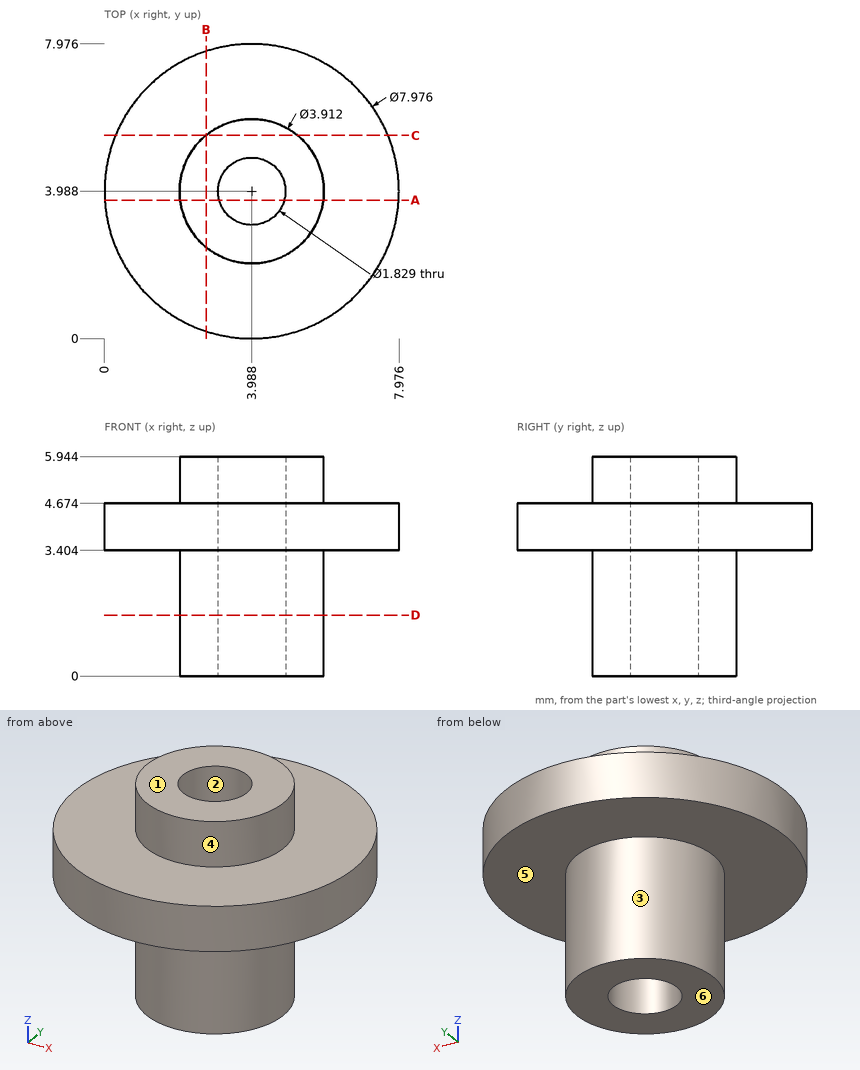
Part print with two shaded views. Sizes in mm from the minimum x, y, z corner. A direction names the side the tool comes from. Round coordinates to 2 decimals unless told otherwise and drop trailing zeros. Order: outer loops, then holes, each group sorted by start corner. A loop starts at its lowest first (then second) coordinate and runs counter-clockwise, first axis right, second up. Notation, with made-up numbers: (-12.75, 41) - (18.25, 41) arc R28 ccw to (18.25, 74) - close; hole circle Ø3 at (-30, 75). An arc over 180 degrees is marked (long way). Answer as CSV lines item,"result". Start each with the question number.
1. Drill centre lines: L1, parallel to X at y = 4, z = 5.55; L2, parallel to Z at x = 2, y = 1.75; L3, parallel to Y at x = 4.75, z = 5.55 (1 decimal). Where is each one in solid material? Low to high. Write a range as [from, to].
2. Pull direction X, two halves, no side cores. Call the marked faces 1, 2 and 3: +X half, -X half, draft (parallel to the pull), parting line (faces both ways), or undercut.
3. Saw through at B-B, the plane x = 2.75. Write the cut outline in (y, z).
4. Saw through at A-A, the plane y = 3.75. Write the cut outline in (x, z) (1 decimal).
5. Saw through at D-D, the plane z = 1.65. Write the cut outline in (x, y) (1 decimal).
6. Saw through at C-C, the plane y = 5.5. Write the cut outline in (x, z).
7. Pin check, flat tips, straight feed: pin 1 (2 mm diameter, centred on x = 7, z = 4.5, fed in from +Y); pin 2 (1.5 mm diameter, centred on x = 2, y = 1, fed in from -Z). Stop position of each tip, or through.
8. Tool access for the marked faces 4, 5 and 6: list every direction of +Z, -Z, +X, -X, +Y, -Y with a clear straight run to the whole face (end or side of a thin tool).
Model answer:
1,L1,"x = [2.03, 3.07], [4.9, 5.94]"
1,L2,"z = [3.4, 4.67]"
1,L3,"y = [2.2, 3.5], [4.5, 5.8]"
2,face 1,"draft"
2,face 2,"undercut"
2,face 3,"parting line"
3,outline,"(0.2, 3.4) - (2.47, 3.4) - (2.47, 0) - (5.5, 0) - (5.5, 3.4) - (7.78, 3.4) - (7.78, 4.67) - (5.5, 4.67) - (5.5, 5.94) - (2.47, 5.94) - (2.47, 4.67) - (0.2, 4.67) - close"
4,outline,"(0, 3.4) - (2, 3.4) - (2, 0) - (3.1, 0) - (3.1, 5.9) - (2, 5.9) - (2, 4.7) - (0, 4.7) - close; (4.9, 0) - (5.9, 0) - (5.9, 3.4) - (8, 3.4) - (8, 4.7) - (5.9, 4.7) - (5.9, 5.9) - (4.9, 5.9) - close"
5,outline,"circle Ø3.9 at (4, 4); hole circle Ø1.8 at (4, 4)"
6,outline,"(0.3, 3.4) - (2.75, 3.4) - (2.75, 0) - (5.23, 0) - (5.23, 3.4) - (7.68, 3.4) - (7.68, 4.67) - (5.23, 4.67) - (5.23, 5.94) - (2.75, 5.94) - (2.75, 4.67) - (0.3, 4.67) - close"
7,pin 1,"stops at y = 7.43"
7,pin 2,"stops at z = 3.4"
8,face 4,"+Z"
8,face 5,"-Z"
8,face 6,"-Z, +X, -X, +Y, -Y"
